Here's how the part is built. I have some questions about the finished solid (model axes, mm). Face numbers are marked on the shaded views. A direction names the side the tool comes from. Give positions to 0.01 mm unless a question says otherwise; leave off trailing zeros. Loops run counter-clockwise (first coordinate to the right, second up) from the corner with the lowest first, then second, coordinate; pieces in that order, holes last.
Q1. I need wall thicknesses on probe 1 along Z at (x, y) = (48.3, 8.5); probe 2 along X at (y, z) = (10, 72.5). Which ranges of each line are inside material? Lowest first, please.
Q2. For the marked faces 1 and 2, which set-ups out of +Z, -Z, +X, -X, +Y, -Y let a thin tool reach every point of the face, with its end or its side?
Q3. Suppose I cut it at C-C (x = 35). List the corners of the cut face in (y, z) for me, and give its area (3 significant figures).
Q4. Suppose I cut it at A-A (y = 0). List the corners of the cut face in (x, z) for me.
Q5. Suppose I cut it at D-D (y = 41). List the corners of the cut face in (x, z) for me.
Q6. Thinking about a two-plate mould opening in X: for the marked faces 3, 4, 5 and 6, which applies, pulls with the +X half, pulls with the -X half, needs draft (parallel to the pull), parting line crosses it, or undercut?
Q7. Suppose I cut it at B-B (z = 125). List the corners of the cut face in (x, y) for me.
Q8. I'm going to push flat-ended pins straight in: P1, Ø16, axis at y = -31, z = 44, coming from the +X side; P2, Ø5.5, axis at y = 35, z = 56, coming from the -X side. Where does each tip first touch, or does it pass through?
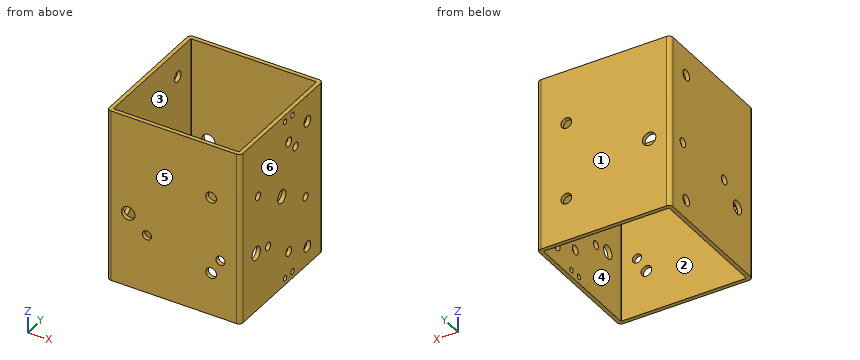
```python
from build123d import *

# Parameters (mm, degrees)
SKETCH1_W                      = 100
SKETCH1_H                      = 100
SKETCH1_W_2                    = 94
SKETCH1_H_2                    = 94
EXTRUDE_THIN1_DEPTH            = 130
FILLET1_R                      = 0.5
FILLET2_R                      = 3
F_8_0_8_DIAMETER_HOLE2_D       = 8
F_8_0_8_DIAMETER_HOLE3_D       = 8
F_10_0_10_DIAMETER_HOLE1_D     = 10
F_10_0_10_DIAMETER_HOLE2_D     = 10
M8X1_25_TAPPED_HOLE1_D         = 6.8
M8X1_25_TAPPED_HOLE1_DEPTH     = 3
M8X1_25_TAPPED_HOLE2_D         = 6.8
M8X1_25_TAPPED_HOLE2_DEPTH     = 3
F_10_0_10_DIAMETER_HOLE3_D     = 10
F_10_0_10_DIAMETER_HOLE3_DEPTH = 3
F_6_0_6_DIAMETER_HOLE1_D       = 6
F_6_0_6_DIAMETER_HOLE1_DEPTH   = 3
CUT_EXTRUDE1_REACH             = 173.464
SKETCH27_R                     = 2
SKETCH27_R_2                   = 3.5


with BuildPart() as part:
    # Sketch1 → Extrude-Thin1 (new body)
    with BuildSketch(Plane.XY):
        Rectangle(SKETCH1_W, SKETCH1_H)
        Rectangle(SKETCH1_W_2, SKETCH1_H_2, mode=Mode.SUBTRACT)
    extrude(amount=EXTRUDE_THIN1_DEPTH)

    # Fillet1
    fillet1_edges = [part.edges().sort_by_distance(p)[0] for p in [
        (47, -47, 65),
        (47, 47, 65),
        (-47, 47, 65),
        (-47, -47, 65),
    ]]
    fillet(fillet1_edges, radius=FILLET1_R)

    # Fillet2
    fillet2_edges = [part.edges().sort_by_distance(p)[0] for p in [
        (50, -50, 65),
        (-50, -50, 65),
        (-50, 50, 65),
        (50, 50, 65),
    ]]
    fillet(fillet2_edges, radius=FILLET2_R)

    # Ø8.0 (8) Diameter Hole2 (through all)
    with Locations(Plane(origin=(0, 50, 0), x_dir=(1, 0, 0), z_dir=(0, 1, 0))):
        with Locations((28, -32), (28, -90)):
            Hole(F_8_0_8_DIAMETER_HOLE2_D / 2)

    # Ø8.0 (8) Diameter Hole3 (through all)
    with Locations(Plane(origin=(50, 0, 0), x_dir=(0, 0, -1), z_dir=(1, 0, 0))):
        with Locations((-14, 31), (-110, 31)):
            Hole(F_8_0_8_DIAMETER_HOLE3_D / 2)

    # Ø10.0 (10) Diameter Hole1 (through all)
    with Locations(Plane(origin=(0, 50, 0), x_dir=(1, 0, 0), z_dir=(0, 1, 0))):
        with Locations((-34, -56)):
            Hole(F_10_0_10_DIAMETER_HOLE1_D / 2)

    # Ø10.0 (10) Diameter Hole2 (through all)
    with Locations(Plane(origin=(50, 0, 0), x_dir=(0, 0, -1), z_dir=(1, 0, 0))):
        with Locations((-44, -31)):
            Hole(F_10_0_10_DIAMETER_HOLE2_D / 2)

    # M8x1.25 Tapped Hole1
    with Locations(Plane.ZY.offset(50)):
        with Locations((56, -15), (56, 35)):
            Hole(M8X1_25_TAPPED_HOLE1_D / 2, depth=M8X1_25_TAPPED_HOLE1_DEPTH)

    # M8x1.25 Tapped Hole2
    with Locations(Plane(origin=(0, -50, 0), x_dir=(-1, 0, 0), z_dir=(0, -1, 0))):
        with Locations((20, -44), (-35, -44)):
            Hole(M8X1_25_TAPPED_HOLE2_D / 2, depth=M8X1_25_TAPPED_HOLE2_DEPTH)

    # Ø10.0 (10) Diameter Hole3
    with Locations(Plane(origin=(50, 0, 0), x_dir=(0, 0, -1), z_dir=(1, 0, 0))):
        with Locations((-70, 0)):
            Hole(F_10_0_10_DIAMETER_HOLE3_D / 2, depth=F_10_0_10_DIAMETER_HOLE3_DEPTH)

    # Ø6.0 (6) Diameter Hole1
    with Locations(Plane(origin=(50, 0, 0), x_dir=(0, 0, -1), z_dir=(1, 0, 0))):
        with Locations((-41.157258279, -16.652364697), (-53.347635303, 28.842741721), (-98.842741721, 16.652364697), (-86.652364697, -28.842741721)):
            Hole(F_6_0_6_DIAMETER_HOLE1_D / 2, depth=F_6_0_6_DIAMETER_HOLE1_DEPTH)

    # Sketch27 → Cut-Extrude1 (cut, up to next)
    with BuildSketch(Plane(origin=(50, 0, 0), x_dir=(0, 0, -1), z_dir=(1, 0, 0)), mode=Mode.PRIVATE) as cut_extrude1_sk1:
        with Locations(Location((-5, 13, 0), (0, 0, 90))):
            Circle(SKETCH27_R)
    cut_extrude1_tool1 = extrude(cut_extrude1_sk1.sketch, amount=-CUT_EXTRUDE1_REACH, mode=Mode.PRIVATE) & part.part
    # Sketch27 → Cut-Extrude1 (cut, up to next)
    with BuildSketch(Plane(origin=(50, 0, 0), x_dir=(0, 0, -1), z_dir=(1, 0, 0)), mode=Mode.PRIVATE) as cut_extrude1_sk2:
        with Locations(Location((-5, 4, 0), (0, 0, 90))):
            Circle(SKETCH27_R)
    cut_extrude1_tool2 = extrude(cut_extrude1_sk2.sketch, amount=-CUT_EXTRUDE1_REACH, mode=Mode.PRIVATE) & part.part
    # Sketch27 → Cut-Extrude1 (cut, up to next)
    with BuildSketch(Plane(origin=(50, 0, 0), x_dir=(0, 0, -1), z_dir=(1, 0, 0)), mode=Mode.PRIVATE) as cut_extrude1_sk3:
        with Locations(Location((-23, 8.5, 0), (0, 0, 90))):
            Circle(SKETCH27_R_2)
    cut_extrude1_tool3 = extrude(cut_extrude1_sk3.sketch, amount=-CUT_EXTRUDE1_REACH, mode=Mode.PRIVATE) & part.part
    # Sketch27 → Cut-Extrude1 (cut, up to next)
    with BuildSketch(Plane(origin=(50, 0, 0), x_dir=(0, 0, -1), z_dir=(1, 0, 0)), mode=Mode.PRIVATE) as cut_extrude1_sk4:
        with Locations(Location((-107, 8.5, 0), (0, 0, 270))):
            Circle(SKETCH27_R_2)
    cut_extrude1_tool4 = extrude(cut_extrude1_sk4.sketch, amount=-CUT_EXTRUDE1_REACH, mode=Mode.PRIVATE) & part.part
    # Sketch27 → Cut-Extrude1 (cut, up to next)
    with BuildSketch(Plane(origin=(50, 0, 0), x_dir=(0, 0, -1), z_dir=(1, 0, 0)), mode=Mode.PRIVATE) as cut_extrude1_sk5:
        with Locations(Location((-125, 4, 0), (0, 0, 270))):
            Circle(SKETCH27_R)
    cut_extrude1_tool5 = extrude(cut_extrude1_sk5.sketch, amount=-CUT_EXTRUDE1_REACH, mode=Mode.PRIVATE) & part.part
    # Sketch27 → Cut-Extrude1 (cut, up to next)
    with BuildSketch(Plane(origin=(50, 0, 0), x_dir=(0, 0, -1), z_dir=(1, 0, 0)), mode=Mode.PRIVATE) as cut_extrude1_sk6:
        with Locations(Location((-125, 13, 0), (0, 0, 270))):
            Circle(SKETCH27_R)
    cut_extrude1_tool6 = extrude(cut_extrude1_sk6.sketch, amount=-CUT_EXTRUDE1_REACH, mode=Mode.PRIVATE) & part.part
    add(cut_extrude1_tool1.solids().sort_by_distance((50, 13, 5))[0], mode=Mode.SUBTRACT)
    add(cut_extrude1_tool2.solids().sort_by_distance((50, 4, 5))[0], mode=Mode.SUBTRACT)
    add(cut_extrude1_tool3.solids().sort_by_distance((50, 8.5, 23))[0], mode=Mode.SUBTRACT)
    add(cut_extrude1_tool4.solids().sort_by_distance((50, 8.5, 107))[0], mode=Mode.SUBTRACT)
    add(cut_extrude1_tool5.solids().sort_by_distance((50, 4, 125))[0], mode=Mode.SUBTRACT)
    add(cut_extrude1_tool6.solids().sort_by_distance((50, 13, 125))[0], mode=Mode.SUBTRACT)


solid = part.part
```
Solutions:
1. probe 1: z = 0 to 19.5, 26.5 to 103.5, 110.5 to 130
1. probe 2: x = -50 to -47, 47 to 50
2. face 1: +Z, -Z, +X, -X, +Y
2. face 2: +Z, -Z
3. outline: (-50, 0) - (-47, 0) - (-47, 40.6) - (-50, 40.6) - close; (-50, 47.4) - (-47, 47.4) - (-47, 130) - (-50, 130) - close; (47, 0) - (50, 0) - (50, 130) - (47, 130) - close
3. area: 760 mm2
4. outline: (-50, 0) - (-47, 0) - (-47, 130) - (-50, 130) - close; (47, 0) - (50, 0) - (50, 65) - (47, 65) - close; (47, 75) - (50, 75) - (50, 130) - (47, 130) - close
5. outline: (-50, 0) - (-47, 0) - (-47, 130) - (-50, 130) - close; (47, 0) - (50, 0) - (50, 130) - (47, 130) - close
6. face 3: undercut
6. face 4: undercut
6. face 5: needs draft
6. face 6: pulls with the +X half
7. outline: (-50, -47) arc R3 ccw to (-47, -50) - (47, -50) arc R3 ccw to (50, -47) - (50, 2) - (47, 2) - (47, -46.5) arc R0.5 cw to (46.5, -47) - (-46.5, -47) arc R0.5 cw to (-47, -46.5) - (-47, 46.5) arc R0.5 cw to (-46.5, 47) - (46.5, 47) arc R0.5 cw to (47, 46.5) - (47, 15) - (50, 15) - (50, 47) arc R3 ccw to (47, 50) - (-47, 50) arc R3 ccw to (-50, 47) - close; (47, 6) - (50, 6) - (50, 11) - (47, 11) - close
8. P1: stops at x = 50
8. P2: stops at x = 47
